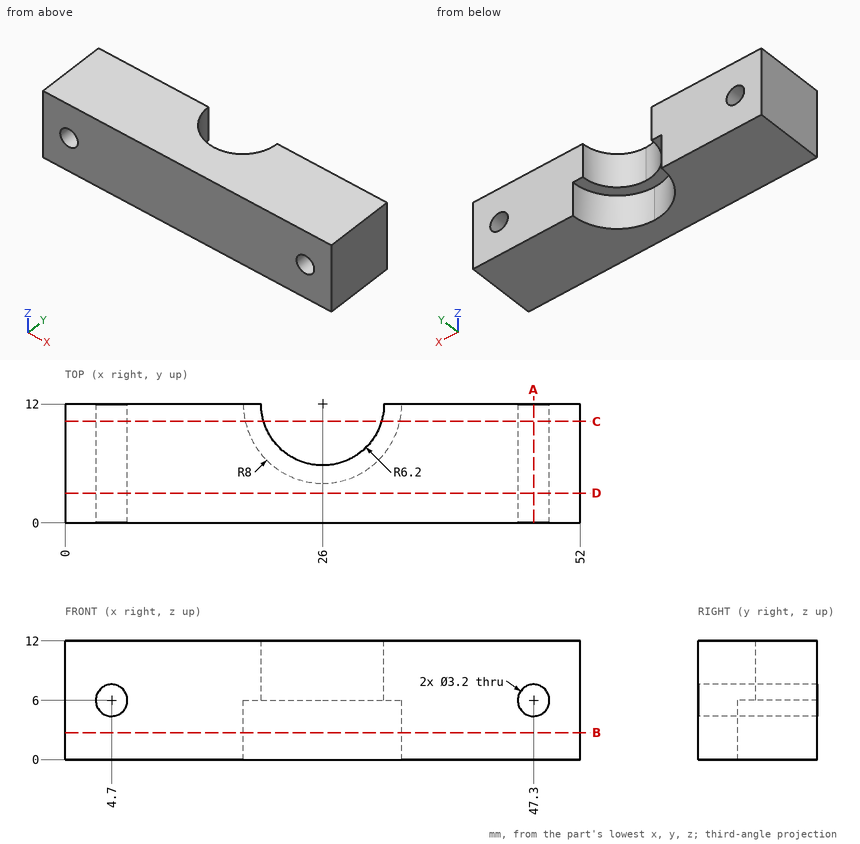
Verification items for this drawing (mm, ordinates from the low corner). Give positions to 0.01 mm unless a question says otherwise; leave off trailing zeros. Write each loop counter-clockwise with the first axis right and the second up, starting at its lowest first coordinate (ties: lowest second). Pieces come first, ordered by that corner, then holes.
1) Section check C-C, the plane y = 10.25. Record the boundary of the cut face in (x, z), and give its area (3 significant figures).
2) Section check D-D, the plane y = 3. Record the boundary of the cut face in (x, z), and give its area (3 significant figures).
3) Material ranges on L1, parallel to Z at x = 4.7, y = 7.5; L2, parallel to X at y = 3.5, z = 5; L3, parallel to X at y = 8.75, z = 2.75, recorded low to high.
4) Gauge pin test, flat end, axial feed: pin 1 (2.5 mm diameter, centred on x = 27.5, y = 6.5, fed in from -Z). Record the tip position at first contact, or that the pin passes through.
5) Section check A-A, the plane x = 47.3. Record the boundary of the cut face in (y, z), and give its area (3 significant figures).
6) Section check B-B, the plane z = 2.75. Record the boundary of the cut face in (x, y).
Computed:
1. outline: (0, 0) - (18.19, 0) - (18.19, 6) - (20.05, 6) - (20.05, 12) - (0, 12) - close; (31.95, 6) - (33.81, 6) - (33.81, 0) - (52, 0) - (52, 12) - (31.95, 12) - close; hole circle Ø3.2 at (4.7, 6); hole circle Ø3.2 at (47.3, 6)
1. area: 443 mm2
2. outline: (0, 0) - (52, 0) - (52, 12) - (0, 12) - close; hole circle Ø3.2 at (4.7, 6); hole circle Ø3.2 at (47.3, 6)
2. area: 608 mm2
3. L1: z = 0 to 4.4, 7.6 to 12
3. L2: x = 0 to 3.45, 5.95 to 46.05, 48.55 to 52
3. L3: x = 0 to 18.69, 33.31 to 52
4. pin 1: stops at z = 6
5. outline: (0, 0) - (12, 0) - (12, 4.4) - (0, 4.4) - close; (0, 7.6) - (12, 7.6) - (12, 12) - (0, 12) - close
5. area: 106 mm2
6. outline: (0, 0) - (52, 0) - (52, 12) - (34, 12) arc R8 cw to (26, 4) arc R8 cw to (18, 12) - (0, 12) - close
